Work out the finished part from the listing and answer in its coordinate system (mm). A direction names the side the tool comes from. Give positions to 0.01 mm unless a question says otherwise; leave off trailing zeros. Loops run counter-clockwise (first coordinate to the right, second up) from the corner with the lowest first, then second, coordinate; pieces in that order, holes last. Notation, with made-up numbers: M 15,8 L 25,8 A11 cw 25,15 Z; hole C 1.5,34.25 d7. An arc over 180 degrees is marked long. Write item = value, one per line. Start each with the question number.
1. Section C-C on x = -34.5 is taken. Determine the outline of the cut face in (y, z).
2. For faces 1 (the face through (49, -17, 0)), 2 (the face through (-97.5, 5.1, 0.5)), determine the directions among +Z, -Z, +X, -X, +Y, -Y from which every point of the face is accessible in a straight line to the end or side of a thin tool.
3. Section D-D on z = -8.75 is taken. Determine the outline of the cut face in (x, y), plus the area to 3 significant figures.
4. Section A-A on y = -30 is taken. Determine the outline of the cut face in (x, z), plus the area to 3 significant figures.
5. Consider L1, parallel to X at y = 5.5, z = 0.5; L2, parallel to X at y = -20.5, z = -5.5; L3, parallel to X at y = -36, z = -11.5. Determine where each line is inside the solid, lowest interval first. Write a range as [from, to].
6. The mould has two halves that part along X. Classify faces 3 (the face through (57.096, -48.515, -5.754)), 4 (the face through (-51, -17, 0)), 5 (the face through (-1, -20, 1)): released by +X, released by -X, zero draft, split by the parting line, or undercut.
7. Flat-ended cylindrical pins translate along their axes: pin 1 Ø16.5 at (x, y) = (39, -18.5) entering from -Z; pin 2 Ø8 at (y, z) = (-20, -7) entering from -X; pin 3 Ø6 at (x, z) = (-24.5, -10.5) entering from +Y. Find the tip coordinate at first contact, or state that the pin passes through.
8. Section B-B on y = -11 is taken. Determine the outline of the cut face in (x, z) (3 decimals).
```python
from build123d import *

# Parameters (mm, degrees)
SKETCH_R     = 2.5
PAD_DEPTH    = 1
PAD001_DEPTH = 12.7


with BuildPart() as part:
    # Sketch → Pad (new body)
    with BuildSketch(Plane.XY):
        with BuildLine():
            ThreePointArc((0, -21.794495), (56.18034, -48.733972), (95, 0))
            ThreePointArc((95, 0), (98.535534, 8.535534), (90, 5))
            Line((90, 5), (90, 0))
            Line((-90, 0), (90, 0))
            Line((-90, 5), (-90, 0))
            ThreePointArc((-90, 5), (-98.535534, 8.535534), (-95, 0))
            ThreePointArc((-95, 0), (-56.18034, -48.733972), (0, -21.794495))
        make_face()
        with Locations((95, 5)):
            Circle(SKETCH_R, mode=Mode.SUBTRACT)
        with Locations((-95, 5)):
            Circle(SKETCH_R, mode=Mode.SUBTRACT)
    extrude(amount=PAD_DEPTH)

    # Sketch001 (on Face10 of Pad) → Pad001 (join)
    with BuildSketch(Plane(origin=(0, 0, 0), x_dir=(1, 0, 0), z_dir=(0, 0, -1))):
        with BuildLine():
            Line((-95, 0), (-85.5, 19.615045))
            ThreePointArc((0, 0), (-34.937694, 43.860575), (-85.5, 19.615045))
            ThreePointArc((85.5, 19.615045), (34.937694, 43.860575), (0, 0))
            Line((95, 0), (85.5, 19.615045))
            ThreePointArc((95, 0), (56.18034, 48.733972), (0, 21.794495))
            ThreePointArc((0, 21.794495), (-56.18034, 48.733972), (-95, 0))
        make_face()
    extrude(amount=PAD001_DEPTH)


solid = part.part
```
Verdict:
q1.outline = M -48.89,-12.7 L -43.76,-12.7 L -43.76,0 L 0,0 L 0,1 L -48.89,1 Z
q2.face_1 = -Z, +Y
q2.face_2 = +Z, -Z
q3.outline = M -95,0 A50 ccw 0,-21.79 A50 ccw 95,0 L 85.5,-19.62 A45 cw 0,0 A45 cw -85.5,-19.62 Z
q3.area = 1,280 mm2
q4.outline = M -85,-12.7 L -78.54,-12.7 L -78.54,0 L -11.46,0 L -11.46,-12.7 L -5,-12.7 L -5,1 L -85,1 Z; M 5,-12.7 L 11.46,-12.7 L 11.46,0 L 78.54,0 L 78.54,-12.7 L 85,-12.7 L 85,1 L 5,1 Z
q4.area = 488 mm2
q5.L1 = [-99.97, -97.45], [-92.55, -90.03], [90.03, 92.55], [97.45, 99.97]
q5.L2 = [-90.6, -85.06], [-4.94, 4.94], [85.06, 90.6]
q5.L3 = [-79.7, -72], [-18, -10.3], [10.3, 18], [72, 79.7]
q6.face_3 = undercut
q6.face_4 = undercut
q6.face_5 = zero draft
q7.pin_1 = 0
q7.pin_2 = -92.37
q7.pin_3 = -38.38
q8.outline = M -93.775,-12.7 L -89.672,-12.7 L -89.672,0 L -1.365,0 L -1.365,-12.7 L 1.365,-12.7 L 1.365,0 L 89.672,0 L 89.672,-12.7 L 93.775,-12.7 L 93.775,1 L -93.775,1 Z
